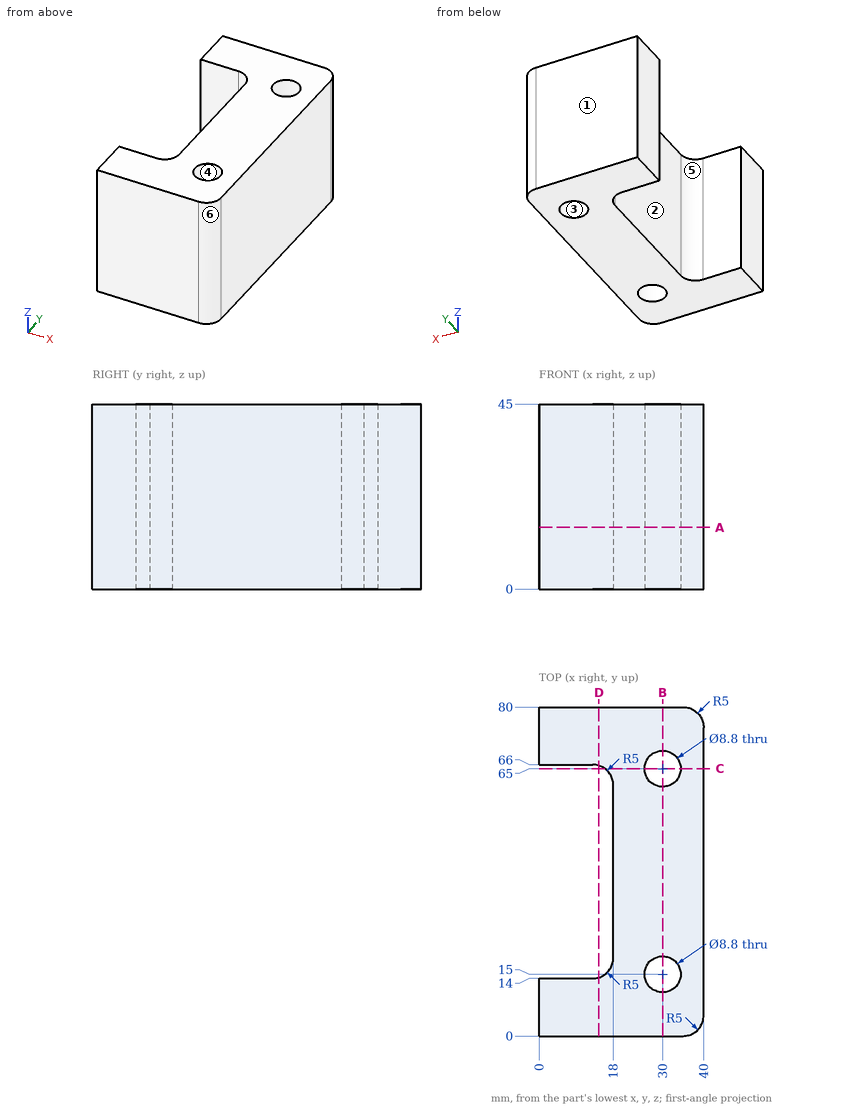
Verification items for this drawing (mm, ordinates from the low corner). A direction names the side the tool comes from. Round coordinates to 2 decimals unless told otherwise and drop trailing zeros. Write each loop counter-clockwise with the first axis right and the second up, starting at its lowest first coordinate (ties: lowest second). Pieces come first, ordered by that corner, then holes. Notation, with made-up numbers: M 1.25,79 L 42.25,79 A38 cw 42.25,117 Z; hole C 40.25,51 d10. An arc over 180 degrees is marked long. Write item = value, one per line. Start each with the question number.
1. Section check A-A, the plane z = 15. Record the cut outline in (x, y), then the cut area to 3 significant figures.
2. Section check C-C, the plane y = 65. Record the cut outline in (x, z), then the cut area to 3 significant figures.
3. Release check for a two-part mould opening along X. For the marked faces 1, 2, 3 and 4 record: pulls with the +X half, pulls with the -X half, needs draft (parallel to the pull), parting line crosses it, or undercut.
4. Tool access check on the marked faces 5 and 6. Record the directions out of +Z, -Z, +X, -X, +Y, -Y that give a thin tool (end or side, any length) a straight path to the whole face; none if there is none.
5. Section check B-B, the plane x = 30. Record the cut outline in (y, z), then the cut area to 3 significant figures.
6. Section check D-D, the plane x = 14.5. Record the cut outline in (y, z), then the cut area to 3 significant figures.
7. Gauge pin test, flat ends, axial feed: pin 1 (8 mm diameter, centred on y = 20.5, z = 20.5, fed in from -X); pin 2 (12.5 mm diameter, centred on y = 44, z = 27, fed in from -X); pin 3 (8 mm diameter, centred on x = 30, y = 65, fed in from -Z). Record the tip position at first contact, or that the pin passes through.
8. Scan lines: line 1 (Y direction, x = 30, z = 35); line 2 (Y direction, x = 14, z = 5); line 3 (Y direction, x = 13.5, z = 33.5). Record each from-to range of solid material in increasing order. Write a range as [from, to].
Results found:
q1.outline = M 0,0 L 35,0 A5 ccw 40,5 L 40,75 A5 ccw 35,80 L 0,80 L 0,66 L 13,66 A5 cw 18,61 L 18,19 A5 cw 13,14 L 0,14 Z; hole C 30,15 d8.8; hole C 30,65 d8.8
q1.area = 2,140 mm^2
q2.outline = M 16,0 L 25.6,0 L 25.6,45 L 16,45 Z; M 34.4,0 L 40,0 L 40,45 L 34.4,45 Z
q2.area = 684 mm^2
q3.face_1 = needs draft
q3.face_2 = pulls with the -X half
q3.face_3 = undercut
q3.face_4 = undercut
q4.face_5 = +Z, -Z, -X
q4.face_6 = +Z, -Z, +X, -Y
q5.outline = M 0,0 L 10.6,0 L 10.6,45 L 0,45 Z; M 19.4,0 L 60.6,0 L 60.6,45 L 19.4,45 Z; M 69.4,0 L 80,0 L 80,45 L 69.4,45 Z
q5.area = 2,810 mm^2
q6.outline = M 0,0 L 14.23,0 L 14.23,45 L 0,45 Z; M 65.77,0 L 80,0 L 80,45 L 65.77,45 Z
q6.area = 1,280 mm^2
q7.pin_1 = 17.33
q7.pin_2 = 18
q7.pin_3 = through
q8.line_1 = [0, 10.6], [19.4, 60.6], [69.4, 80]
q8.line_2 = [0, 14.1], [65.9, 80]
q8.line_3 = [0, 14.03], [65.97, 80]
